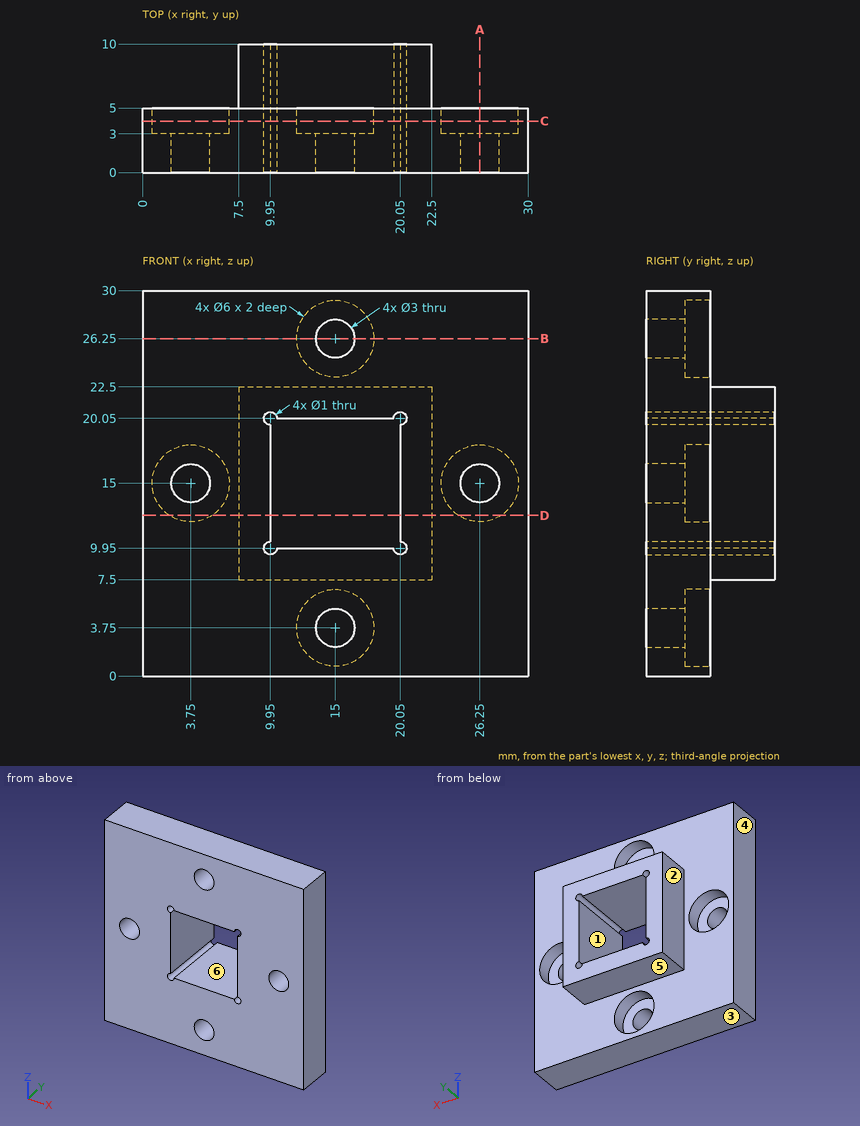
For this review, use the dimensioned drawing (mm, ordinates from the lowest corner) and the shaded views. A direction names the side the tool comes from. Coordinates: 2 decimals unless noted, no trailing zeros. Loops run counter-clockwise (first coordinate to the right, second up) from the corner with the lowest first, then second, coordinate; pieces in that order, holes last.
1. For the marked faces 1, 2 and 3, list the 3-axis set-ups (+Z, -Z, +X, -X, +Y, -Y) from which the entire face can be reached by the end or side of a thin tool; tool diameter is ignored.
2. Mouldability with a two-part tool opening along Z and no side actions: class the marked faces 4, 5 and 6 as +Z half, -Z half, draft (parallel to the pull), parting line (faces both ways), or undercut.
3. Insertion check: P1, Ø9.5, axis at x = 3.75, z = 15, coming from the -Y side; P2, Ø3.5, axis at x = 15, z = 26.25, coming from the +Y side; P3, Ø5.5, axis at y = 8.5, z = 14.5, coming from the +X side; P4, Ø1.5, axis at y = 9, z = 21.5, coming from the -X side. Each pin has a flat end and moves straight along its axis. Give the tip position at first contact, or say it passes through.
4. Add section D-D, the plane z = 12.5. Give the boundary of the cut face in (x, y).
5. For line 1 (X direction, y = 4.5, z = 15); line 2 (Y direction, x = 5.25, z = 25); line 3 (Z direction, x = 14, y = 0.5), list the stretches that pass through material, from the lowest coordinate up.
6. Add section C-C, the plane y = 4. Give the boundary of the cut face in (x, z), then the cut area to 3 significant figures.
7. Add section A-A, the plane x = 26.25. Give the boundary of the cut face in (y, z), then the cut area to 3 significant figures.
8. Add section B-B, the plane z = 26.25. Give the boundary of the cut face in (x, y), then the cut area to 3 significant figures.
Result:
1. face 1: +Y, -Y
1. face 2: +Z, -Z, -X, +Y
1. face 3: -Z, +X, -X, +Y, -Y
2. face 4: draft
2. face 5: -Z half
2. face 6: undercut
3. P1: stops at y = 0
3. P2: stops at y = 3
3. P3: stops at x = 22.5
3. P4: stops at x = 7.5
4. outline: (0, 0) - (9.95, 0) - (9.95, 10) - (7.5, 10) - (7.5, 5) - (5.41, 5) - (5.41, 3) - (2.09, 3) - (2.09, 5) - (0, 5) - close; (20.05, 0) - (30, 0) - (30, 5) - (27.91, 5) - (27.91, 3) - (24.59, 3) - (24.59, 5) - (22.5, 5) - (22.5, 10) - (20.05, 10) - close
5. line 1: x = 0 to 0.75, 6.75 to 9.95, 20.05 to 23.25, 29.25 to 30
5. line 2: y = 0 to 5
5. line 3: z = 0 to 2.63, 4.87 to 9.95, 20.05 to 25.13, 27.37 to 30
6. outline: (0, 0) - (30, 0) - (30, 30) - (0, 30) - close; hole circle Ø6 at (3.75, 15); hole (9.95, 10.45) arc R0.5 ccw (long way) to (10.45, 9.95) - (19.55, 9.95) arc R0.5 ccw (long way) to (20.05, 10.45) - (20.05, 19.55) arc R0.5 ccw (long way) to (19.55, 20.05) - (10.45, 20.05) arc R0.5 ccw (long way) to (9.95, 19.55) - close; hole circle Ø6 at (15, 3.75); hole circle Ø6 at (15, 26.25); hole circle Ø6 at (26.25, 15)
6. area: 683 mm2
7. outline: (0, 0) - (5, 0) - (5, 12) - (3, 12) - (3, 13.5) - (0, 13.5) - close; (0, 16.5) - (3, 16.5) - (3, 18) - (5, 18) - (5, 30) - (0, 30) - close
7. area: 129 mm2
8. outline: (0, 0) - (13.5, 0) - (13.5, 3) - (12, 3) - (12, 5) - (0, 5) - close; (16.5, 0) - (30, 0) - (30, 5) - (18, 5) - (18, 3) - (16.5, 3) - close
8. area: 129 mm2
